Autodesk Inventor part; units mm, degrees
sketch "Sketch1" plane through (0, 0, 0) normal (0, 0, 1) x (1, 0, 0)
  line L0 (0, 2.8582) -> (0, -2.8582) construction
  line L1 (-5.7775, 0) -> (5.7775, 0) construction
  line L2 (-75, -137.5) -> (75, -137.5)
  line L3 (75, -137.5) -> (75, 137.5)
  line L4 (75, 137.5) -> (-75, 137.5)
  line L5 (-75, 137.5) -> (-75, -137.5)
  line L6 (-75, -137.5) -> (75, 137.5) construction
  line L7 (75, -137.5) -> (-75, 137.5) construction
  point P0 (0, 0)
  point P1 (0, 0)
  dimension "d0" = 150
  dimension "d1" = 275
extrude "Extrusion1" add sketch "Sketch1" along normal blind 5
sketch "Sketch2" plane through (0, 0, 5) normal (0, 0, 1) x (1, 0, 0)
  line L0 (0, 0) -> (0, -120)
  circle A0 centre (0, -120) radius 5
  line L1 (-75, 137.5) -> (-75, -137.5)
  line L2 (-75, -137.5) -> (-70, -137.5)
  line L3 (-70, -137.5) -> (-70, -92.5)
  line L4 (-70, -92.5) -> (-75, -92.5)
  line L5 (-75, -92.5) -> (-75, -137.5)
  line L6 (-75, -92.5) -> (-75, -77.5)
  line L7 (-75, -77.5) -> (-75, -47.5)
  line L8 (-75, -47.5) -> (-75, -17.5)
  line L9 (-75, -17.5) -> (-75, 12.5)
  line L10 (-75, 12.5) -> (-75, 42.5)
  line L11 (-75, 42.5) -> (-75, 72.5)
  line L12 (-75, 72.5) -> (-75, 102.5)
  line L13 (-75, 102.5) -> (-75, 132.5)
  line L14 (-75, -77.5) -> (-70, -77.5)
  line L15 (-70, -77.5) -> (-70, -47.5)
  line L16 (-70, -47.5) -> (-75, -47.5)
  line L17 (-75, -47.5) -> (-75, -77.5)
  line L18 (-75, -17.5) -> (-70, -17.5)
  line L19 (-70, -17.5) -> (-70, 12.5)
  line L20 (-70, 12.5) -> (-75, 12.5)
  line L21 (-75, 12.5) -> (-75, -17.5)
  line L22 (-75, 42.5) -> (-70, 42.5)
  line L23 (-70, 42.5) -> (-70, 72.5)
  line L24 (-70, 72.5) -> (-75, 72.5)
  line L25 (-75, 72.5) -> (-75, 42.5)
  line L26 (75, 137.5) -> (-75, 137.5)
  line L27 (-75, 102.5) -> (-70, 102.5)
  line L28 (-70, 102.5) -> (-70, 137.5)
  line L29 (-70, 137.5) -> (-75, 137.5)
  line L30 (-75, 137.5) -> (-75, 102.5)
  line L31 (75, -137.5) -> (75, 137.5)
  line L32 (75, -137.5) -> (75, -92.5)
  line L33 (75, -92.5) -> (75, -77.5)
  line L34 (75, -77.5) -> (75, -47.5)
  line L35 (75, -47.5) -> (75, -17.5)
  line L36 (75, -17.5) -> (75, 12.5)
  line L37 (75, 12.5) -> (75, 42.5)
  line L38 (75, 42.5) -> (75, 72.5)
  line L39 (75, 72.5) -> (75, 102.5)
  line L40 (75, 102.5) -> (75, 132.5)
  line L41 (-75, -137.5) -> (75, -137.5)
  line L42 (75, -137.5) -> (70, -137.5)
  line L43 (70, -137.5) -> (70, -92.5)
  line L44 (70, -92.5) -> (75, -92.5)
  line L45 (75, -92.5) -> (75, -137.5)
  line L46 (75, -77.5) -> (70, -77.5)
  line L47 (70, -77.5) -> (70, -47.5)
  line L48 (70, -47.5) -> (75, -47.5)
  line L49 (75, -47.5) -> (75, -77.5)
  line L50 (75, -17.5) -> (70, -17.5)
  line L51 (70, -17.5) -> (70, 12.5)
  line L52 (70, 12.5) -> (75, 12.5)
  line L53 (75, 12.5) -> (75, -17.5)
  line L54 (75, 42.5) -> (70, 42.5)
  line L55 (70, 42.5) -> (70, 72.5)
  line L56 (70, 72.5) -> (75, 72.5)
  line L57 (75, 72.5) -> (75, 42.5)
  line L58 (75, 102.5) -> (70, 102.5)
  line L59 (70, 102.5) -> (70, 137.5)
  line L60 (70, 137.5) -> (75, 137.5)
  line L61 (75, 137.5) -> (75, 102.5)
  line L62 (0, -137.5) -> (-15, -137.5)
  line L63 (-15, -137.5) -> (15, -137.5)
  line L64 (-15, -137.5) -> (-45, -137.5)
  line L65 (-45, -137.5) -> (-45, -132.5)
  line L66 (-45, -132.5) -> (-15, -132.5)
  line L67 (-15, -132.5) -> (-15, -137.5)
  line L68 (15, -137.5) -> (45, -137.5)
  line L69 (45, -137.5) -> (45, -132.5)
  line L70 (45, -132.5) -> (15, -132.5)
  line L71 (15, -132.5) -> (15, -137.5)
  point P0 (-75, -92.5)
  dimension "d4" = 120
  dimension "d5" = 10
  dimension "d6" = 5
  dimension "d7" = 45
  dimension "d9" = 30
  dimension "d10" = 30
  dimension "d11" = 30
  dimension "d12" = 30
  dimension "d13" = 30
  dimension "d14" = 30
  dimension "d15" = 30
  dimension "d16" = 5
  dimension "d17" = 30
  dimension "d18" = 5
  dimension "d19" = 5
  dimension "d20" = 5
  dimension "d21" = 45
  dimension "d23" = 30
  dimension "d24" = 30
  dimension "d25" = 30
  dimension "d26" = 30
  dimension "d27" = 30
  dimension "d28" = 30
  dimension "d29" = 30
  dimension "d30" = 5
  dimension "d31" = 5
  dimension "d32" = 15
  dimension "d33" = 30
  dimension "d34" = 30
  dimension "d35" = 5
  dimension "d36" = 30
  dimension "d37" = 5
  dimension "d40" = 45
extrude "Extrusion2" cut sketch "Sketch2" against normal blind 8 contours A0 | L26 L28 L27 L1 | L26 L31 L58 L59 | L24 L23 L22 L1 | L20 L19 L18 L1 | L31 L54 L55 L56 | L16 L15 L14 L1 | L31 L50 L51 L52 | L4 L3 L2 L1 | L31 L46 L47 L48 | L31 L41 L43 L44 | L65 L66 L67 L41 | L41 L71 L70 L69
sketch "Sketch3" plane through (0, 0, 5) normal (0, 0, 1) x (1, 0, 0)
  line L0 (70, 137.5) -> (-70, 137.5)
  line L1 (0, 137.5) -> (0, 107.5)
  line L2 (0, 107.5) -> (-24.14, 107.5)
  line L3 (0, 107.5) -> (24.14, 107.5)
  line L4 (24.14, 107.5) -> (24.14, 32.57)
  line L5 (-24.14, 107.5) -> (-24.14, 24.95)
  point P0 (0, 0)
  dimension "d42" = 30
  dimension "d43" = 24.14
  dimension "d44" = 24.14
  dimension "d45" = 74.93
  dimension "d46" = 82.55
hole "Hole1" at (-24.14, 24.95, 5) at (24.14, 32.57, 5) at (24.14, 107.5, 5) at (-24.14, 107.5, 5) direction (0, 0, -1) diameter 3.27 end through all
properties part number "Plaat boven" material "S235"
The model under review builds one solid part; all positions refer to its coordinate system, in mm. A direction names the side the tool comes from. Round coordinates to 2 decimals unless told otherwise and drop trailing zeros. Write each loop counter-clockwise with the first axis right and the second up, starting at its lowest first coordinate (ties: lowest second). Pieces come first, ordered by that corner, then holes. Notation, with made-up numbers: (-12.75, -17.5) -> (34.25, -17.5) arc R10 cw to (34.25, -9.5) -> close; hole circle Ø2 at (34.5, 64.25). An arc over 180 degrees is marked (long way). Use CSV: the item, a comma, the result in double quotes.
Q1. For pin 1 Ø2.5 at (x, z) = (-72, 2.5) entering from -Y; pin 2 Ø2.5 at (x, y) = (24.14, 32.57) entering from +Z; pin 3 Ø1.5 at (x, z) = (73, 2.5) entering from +Y; pin 4 Ø2.5 at (y, z) = (-134, 1.5) entering from +X, all flat-tipped, find the tip position at first contact; note any pin that passes through.
Checks:
pin 1,"y = -92.5"
pin 2,"through"
pin 3,"y = 102.5"
pin 4,"x = 70"
Q2. Consider section C-C (y = -54.5). Give the boundary of the cut face in (x, z).
Checks:
outline,"(-70, 0) -> (70, 0) -> (70, 5) -> (-70, 5) -> close"
Q3. Consider section A-A (x = 0). Give the boundary of the cut face in (y, z).
Checks:
outline,"(-137.5, 0) -> (-125, 0) -> (-125, 5) -> (-137.5, 5) -> close; (-115, 0) -> (137.5, 0) -> (137.5, 5) -> (-115, 5) -> close"
Q4. To check wall thickness, follow probe 1 along X at (y, z) = (107.5, 3.85) (3 decimals); probe 2 along Y at (x, z) = (24.14, 3.4) (3 decimals); probe 3 along Y at (x, z) = (-23.5, 3.1). State the ranges of each line that lie inside material, in increasing order. Write a range as [from, to].
Checks:
probe 1,"[-70, -25.775], [-22.505, 22.505], [25.775, 70]"
probe 2,"[-132.5, 30.935], [34.205, 105.865], [109.135, 137.5]"
probe 3,"[-132.5, 23.45], [26.45, 106], [109, 137.5]"
Q5. For faces 1 (the flat face through (70, -115, 3)), 2 (the flat face through (70, 120, 3)), 3 (the flat face through (72, 12.5, 3)), 4 (the flat face through (-72, 12.5, 3)), list the 3-axis set-ups (+Z, -Z, +X, -X, +Y, -Y) from which the entire face can be reached by the end or side of a thin tool; tool diameter is ignored.
Checks:
face 1,"+Z, -Z, +X, -Y"
face 2,"+Z, -Z, +X, +Y"
face 3,"+Z, -Z, +X"
face 4,"+Z, -Z, -X"
Q6. Consider section B-B (z = 3.8). State how many separate pieces and enclosed holes the cut face has, then the cut area to 3 significant figures.
Checks:
separate pieces,"1"
enclosed holes,"5"
area,"39,100 mm²"
Q7. Mouldability with a two-part tool opening along Y and no side actions: class faces 5 (the flat face through (30, -132.5, 3)), 6 (the flat face through (-73, -77.5, 3)), 7 (the flat face through (-45, -135, 3)) as released by +Y, released by -Y, zero draft, split by the parting line, or undercut.
Checks:
face 5,"released by -Y"
face 6,"undercut"
face 7,"zero draft"
Q8. Consider section D-D (x = -39). Give the boundary of the cut face in (y, z), then the cut area to 3 significant figures.
Checks:
outline,"(-132.5, 0) -> (137.5, 0) -> (137.5, 5) -> (-132.5, 5) -> close"
area,"1,350 mm²"
